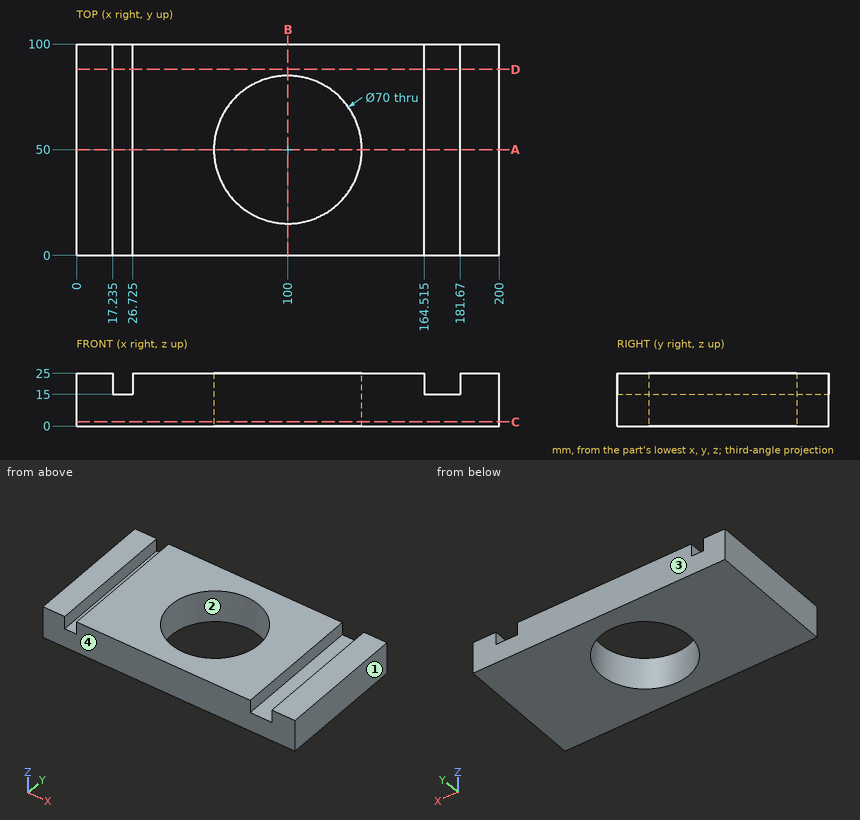
Here's the drawing with two shaded views (mm, measured from the low corner). I have some questions. Coordinates: 2 decimals unless noted, no trailing zeros. Write each loop counter-clockwise with the first axis right and the second up, starting at its lowest first coordinate (ties: lowest second). Pieces come first, ordered by that corner, then holes. Notation, with made-up numbers: (47, -3) -> (66, -3) arc R26 ccw to (66, 27) -> close; hole circle Ø9 at (-26.5, -15). An arc over 180 degrees is marked (long way). Use a Markdown table: item, result. Add a question column.
(1) I'm going to push a flat-ended pin straight in: P1, Ø7.5, axis at x = 24.5, y = 49, coming from the +Z side. Where does the tip first touch, or does it pass through?
(2) If we section it at A-A, the plane y = 50: Write out the boundary of the cut face in (x, z) (1 decimal), and give its area (3 significant figures).
(3) If we section it at B-B, the plane x = 100: Write out the boundary of the cut face in (y, z).
(4) We'd pull the mould along Y, two halves only. Please class the marked faces 1, 2, 3 and 4: +Y half, -Y half, draft (parallel to the pull), parting line (faces both ways), or undercut.
(5) If we section it at D-D, the plane y = 88: Write out the boundary of the cut face in (x, z) (1 decimal), and give its area (3 significant figures).
(6) Please list where these lines run through material, in increasing order: line 1 (X direction, y = 5, z = 16.5) (1 decimal); line 2 (Y direction, x = 100, z = 9); line 3 (X direction, y = 44, z = 18) (1 decimal).
(7) If we section it at C-C, the plane z = 2: Write out the boundary of the cut face in (x, y), and give its area (3 significant figures).
Outcome:
| question | item | result |
|---|---|---|
| 1 | P1 | stops at z = 25 |
| 2 | outline | (0, 0) -> (65, 0) -> (65, 25) -> (26.7, 25) -> (26.7, 15) -> (17.2, 15) -> (17.2, 25) -> (0, 25) -> close; (135, 0) -> (200, 0) -> (200, 25) -> (181.7, 25) -> (181.7, 15) -> (164.5, 15) -> (164.5, 25) -> (135, 25) -> close |
| 2 | area | 2,980 mm^2 |
| 3 | outline | (0, 0) -> (15, 0) -> (15, 25) -> (0, 25) -> close; (85, 0) -> (100, 0) -> (100, 25) -> (85, 25) -> close |
| 4 | face 1 | draft |
| 4 | face 2 | undercut |
| 4 | face 3 | +Y half |
| 4 | face 4 | -Y half |
| 5 | outline | (0, 0) -> (200, 0) -> (200, 25) -> (181.7, 25) -> (181.7, 15) -> (164.5, 15) -> (164.5, 25) -> (26.7, 25) -> (26.7, 15) -> (17.2, 15) -> (17.2, 25) -> (0, 25) -> close |
| 5 | area | 4,730 mm^2 |
| 6 | line 1 | x = 0 to 17.2, 26.7 to 164.5, 181.7 to 200 |
| 6 | line 2 | y = 0 to 15, 85 to 100 |
| 6 | line 3 | x = 0 to 17.2, 26.7 to 65.5, 134.5 to 164.5, 181.7 to 200 |
| 7 | outline | (0, 0) -> (200, 0) -> (200, 100) -> (0, 100) -> close; hole circle Ø70 at (100, 50) |
| 7 | area | 16,200 mm^2 |
